from build123d import *

# Parameters (mm, degrees)
BOSS_EXTRUDE1_DEPTH = 7
BOSS_EXTRUDE3_DEPTH = 10
SKETCH6_R           = 1.35
CUT_EXTRUDE3_DEPTH  = 12
FILLET1_R           = 3.5
FILLET2_R           = 3.5


with BuildPart() as part:
    # Sketch1 → Boss-Extrude1 (new body)
    with BuildSketch(Plane.XY):
        with BuildLine():
            ThreePointArc((5.050452833, -4.633288902), (-0.057176836, -7.835700867), (-5.249547167, -4.77259565))
            Line((-5.249547167, -4.77259565), (-5.181922533, -9.77259565))
            Line((-5.181922533, -9.77259565), (5.118077467, -9.633288902))
            Line((5.118077467, -9.633288902), (5.050452833, -4.633288902))
        make_face()
        with BuildLine():
            ThreePointArc((5.664385761, -2.036231273), (-1.546144107, 3.589638037), (-5.249547167, -4.77259565))
            Line((-5.249547167, -4.77259565), (5.050452833, -4.633288902))
            ThreePointArc((5.050452833, -4.633288902), (5.508816158, -3.370549635), (5.664385761, -2.036231273))
        make_face()
        with BuildLine():
            Line((5.050452833, -4.633288902), (-5.249547167, -4.77259565))
            ThreePointArc((-5.249547167, -4.77259565), (-0.057176836, -7.835700867), (5.050452833, -4.633288902))
        make_face()
    extrude(amount=BOSS_EXTRUDE1_DEPTH)

    # Sketch2 → Boss-Extrude3 (add)
    with BuildSketch(Plane.XY.offset(7)):
        with BuildLine():
            Line((5.063146119, -5.571799449), (5.912597424, -5.560310683))
            ThreePointArc((5.912597424, -5.560310683), (6.622250869, -3.861405013), (6.864385761, -2.036231273))
            ThreePointArc((6.864385761, -2.036231273), (-2.052012342, 4.696332749), (-6.086305185, -5.722594964))
            Line((-6.086305185, -5.722594964), (-5.236853881, -5.711106197))
            Line((-5.236853881, -5.711106197), (-5.249547167, -4.77259565))
            ThreePointArc((-5.249547167, -4.77259565), (-0.214051642, 3.763238321), (5.050452833, -4.633288902))
            Line((5.050452833, -4.633288902), (5.063146119, -5.571799449))
        make_face()
        with BuildLine():
            Line((1.811820806, -5.615773387), (5.063146119, -5.571799449))
            Line((5.063146119, -5.571799449), (5.050452833, -4.633288902))
            ThreePointArc((5.050452833, -4.633288902), (-0.214051642, 3.763238321), (-5.249547167, -4.77259565))
            Line((-5.249547167, -4.77259565), (-5.236853881, -5.711106197))
            Line((-5.236853881, -5.711106197), (-1.985528568, -5.66713226))
            ThreePointArc((-1.985528568, -5.66713226), (-2.264842281, 1.438248968), (3.939385761, -2.036231273))
            ThreePointArc((3.939385761, -2.036231273), (3.367343284, -4.118276805), (1.811820806, -5.615773387))
        make_face()
        with BuildLine():
            Line((5.078495254, -6.706676883), (5.063146119, -5.571799449))
            Line((5.063146119, -5.571799449), (1.811820806, -5.615773387))
            ThreePointArc((1.811820806, -5.615773387), (-0.080505202, -6.110858617), (-1.985528568, -5.66713226))
            Line((-1.985528568, -5.66713226), (-5.236853881, -5.711106197))
            Line((-5.236853881, -5.711106197), (-5.221504746, -6.845983631))
            ThreePointArc((-5.221504746, -6.845983631), (-0.040948408, -9.035591128), (5.078495254, -6.706676883))
        make_face()
        with BuildLine():
            Line((5.118077467, -9.633288902), (5.078495254, -6.706676883))
            ThreePointArc((5.078495254, -6.706676883), (-0.040948408, -9.035591128), (-5.221504746, -6.845983631))
            Line((-5.221504746, -6.845983631), (-5.181922533, -9.77259565))
            Line((-5.181922533, -9.77259565), (5.118077467, -9.633288902))
        make_face()
        with BuildLine():
            Line((5.986984522, -11.060310683), (5.912597424, -5.560310683))
            ThreePointArc((5.912597424, -5.560310683), (5.524642674, -6.154664432), (5.078495254, -6.706676883))
            Line((5.078495254, -6.706676883), (5.118077467, -9.633288902))
            Line((5.118077467, -9.633288902), (-5.181922533, -9.77259565))
            Line((-5.181922533, -9.77259565), (-5.221504746, -6.845983631))
            ThreePointArc((-5.221504746, -6.845983631), (-5.6824181, -6.30623911), (-6.086305185, -5.722594964))
            Line((-6.086305185, -5.722594964), (-6.011918087, -11.222594964))
            Line((-6.011918087, -11.222594964), (5.986984522, -11.060310683))
        make_face()
        with BuildLine():
            ThreePointArc((5.078495254, -6.706676883), (5.524642674, -6.154664432), (5.912597424, -5.560310683))
            Line((5.912597424, -5.560310683), (5.063146119, -5.571799449))
            Line((5.063146119, -5.571799449), (5.078495254, -6.706676883))
        make_face()
        with BuildLine():
            Line((-5.236853881, -5.711106197), (-6.086305185, -5.722594964))
            ThreePointArc((-6.086305185, -5.722594964), (-5.6824181, -6.30623911), (-5.221504746, -6.845983631))
            Line((-5.221504746, -6.845983631), (-5.236853881, -5.711106197))
        make_face()
    extrude(amount=BOSS_EXTRUDE3_DEPTH)

    # Sketch6 → Cut-Extrude3 (cut)
    with BuildSketch(Plane(origin=(0.150657496, -11.139246579, 0), x_dir=(-0.999908551, -0.01352369, 0), z_dir=(0.01352369, -0.999908551, 0))):
        with Locations((0.241163233, -13)):
            Circle(SKETCH6_R)
    extrude(amount=-CUT_EXTRUDE3_DEPTH, mode=Mode.SUBTRACT)

    # Fillet1
    fillet1_edges = [part.edges().sort_by_distance(p)[0] for p in [
        (5.986984522, -11.060310683, 12),
    ]]
    fillet(fillet1_edges, radius=FILLET1_R)

    # Fillet2
    fillet2_edges = [part.edges().sort_by_distance(p)[0] for p in [
        (-6.011918087, -11.222594964, 12),
    ]]
    fillet(fillet2_edges, radius=FILLET2_R)


solid = part.part
The listing builds one solid part. Answer for the finished solid, in the listing's coordinates (mm). A direction names the side the tool comes from. Round coordinates to 2 decimals unless told otherwise and drop trailing zeros. Loops run counter-clockwise (first coordinate to the right, second up) from the corner with the lowest first, then second, coordinate; pieces in that order, holes last. Notation, with made-up numbers: M 22.5,55.25 L 31.5,55.25 A15 ccw 31.5,59.25 Z; hole C 66,47.25 d1. An arc over 180 degrees is marked long. Return JSON: item names as keys, results as strings.
Q1. Find section D-D, the plane z = 2. Determine the outline of the cut face in (x, y), plus the area to 3 significant figures.
Results list:
{"outline": "M -5.25,-4.77 L -5.18,-9.77 L 5.12,-9.63 L 5.05,-4.63 A5.8 ccw long Z", "area": "134 mm2"}
Q2. Find section C-C, the plane x = 3.5. Determine the outline of the cut face in (y, z).
Results list:
{"outline": "M -10.94,7 L -9.66,7 L -9.66,0 L 2.48,0 L 2.48,7 L 3.95,7 L 3.95,17 L -0.2,17 L -0.2,7 L -3.88,7 L -3.88,17 L -10.94,17 Z"}
Q3. Find section A-A, the plane z = 10. Determine the outline of the cut face in (x, y) (3 decimals), plus the area to 3 significant figures.
Results list:
{"outline": "M -6.086,-5.723 L -6.059,-7.723 A3.5 ccw -2.512,-11.175 L 2.487,-11.108 A3.5 ccw 5.94,-7.561 L 5.913,-5.56 A7 ccw long Z; hole C -0.136,-2.036 d8.15", "area": "134 mm2"}
Q4. Each of these flat-tipped pins is pushed along its axis until it touches: pin 1 Ø6 at (y, z) = (-4, 3.5) entering from -X; pin 2 Ø1 at (x, y) = (-2, 0) entering from +Z; pin 3 Ø5 at (y, z) = (-9.5, 9) entering from -X. Where does it stop, or does it pass through?
Results list:
{"pin 1": "stops at x = -5.94", "pin 2": "stops at z = 7", "pin 3": "stops at x = -6.07"}
Q5. Find the intervals of material crossed by line 1 along Y through (x, z) = (-2.5, 14.5); line 2 along Z through (x, y) = (-5.5, -6); line 3 along Z through (x, y) = (-2.5, 0.5), in increasing order. Write a range as from..to.
Results list:
{"line 1": "y = -11.18..-5.36, 1.28..4.55", "line 2": "z = 7..17", "line 3": "z = 0..7"}
Q6. The mould has two halves that part along Y. Classify faces 4 (the face through (-4.973, -10.21, 12.07)), 5 (the face through (0, -7, 17)), 6 (the face through (0.05, -8.53, 11.66)): released by +Y, released by -Y, zero draft, split by the parting line, or undercut.
Results list:
{"face 4": "released by -Y", "face 5": "zero draft", "face 6": "undercut"}
Q7. Which of the six approach directions +Z, -Z, +X, -X, +Y, -Y give full straight-line access (tool end or side, diameter ignored) to faces 1 (the face through (0, -3, 0)), 2 (the face through (-5.4, -4.9, 7)), 3 (the face through (0, -2, 7))?
Results list:
{"face 1": "-Z, +X, -X, +Y, -Y", "face 2": "-Z", "face 3": "+Z"}
Q8. Find section B-B, the plane y = -1.25. Determine the outline of the cut face in (x, z), plus the area to 3 significant figures.
Results list:
{"outline": "M -7.09,7 L -5.88,7 L -5.88,0 L 5.61,0 L 5.61,7 L 6.82,7 L 6.82,17 L 3.86,17 L 3.86,7 L -4.13,7 L -4.13,17 L -7.09,17 Z", "area": "140 mm2"}
